Here's how the part is built. I have some questions about the finished solid (model axes, mm). Coordinates: 2 decimals unless noted, no trailing zeros. Write each loop counter-clockwise with the first axis right and the second up, starting at its lowest first coordinate (ties: lowest second). Pieces come first, ordered by that corner, then holes. Notation, with made-up numbers: (35, -17) -> (87, -17) arc R24 ccw to (87, 15) -> close; hole circle Ø5 at (83.5, 9). An arc over 180 degrees is marked (long way). Put each result on its own line as item: value.
```python
from build123d import *

# Parameters (mm, degrees)
SKETCH1_W           = 28
SKETCH1_H           = 18
BOSS_EXTRUDE2_DEPTH = 1.6
SKETCH4_R           = 0.9
CUT_EXTRUDE5_DEPTH  = 1.6
SKETCH9_R           = 0.4
CUT_EXTRUDE6_DEPTH  = 10


with BuildPart() as part:
    # Sketch1 → Boss-Extrude2 (new body)
    with BuildSketch(Plane(origin=(0, 0, 0), x_dir=(1, 0, 0), z_dir=(0, 1, 0))):
        with Locations((17.78, 7.62)):
            Rectangle(SKETCH1_W, SKETCH1_H)
    extrude(amount=BOSS_EXTRUDE2_DEPTH)

    # Sketch4 → Cut-Extrude5 (cut)
    with BuildSketch(Plane(origin=(0, 0, 0), x_dir=(1, 0, 0), z_dir=(0, 1, 0))):
        with Locations((29.76, 15.24)):
            Circle(SKETCH4_R)
        with Locations((29.76, 0)):
            Circle(SKETCH4_R)
        with Locations((6.32, 0)):
            Circle(SKETCH4_R)
        with Locations((6.32, 15.24)):
            Circle(SKETCH4_R)
    extrude(amount=CUT_EXTRUDE5_DEPTH, mode=Mode.SUBTRACT)

    # Sketch9 → Cut-Extrude6 (cut)
    with BuildSketch(Plane(origin=(0, 0, 0), x_dir=(1, 0, 0), z_dir=(0, 1, 0))):
        with Locations((27.73, 5.42)):
            Circle(SKETCH9_R)
        with Locations((27.73, 9.82)):
            Circle(SKETCH9_R)
    extrude(amount=CUT_EXTRUDE6_DEPTH, mode=Mode.SUBTRACT)


solid = part.part
```
Item 1: Imagine slicing it at C-C on x = 6.32. Write out the boundary of the cut face in (y, z), then the cut area to 3 significant figures.
Output:
outline: (0, -16.62) -> (1.6, -16.62) -> (1.6, -16.14) -> (0, -16.14) -> close; (0, -14.34) -> (1.6, -14.34) -> (1.6, -0.9) -> (0, -0.9) -> close; (0, 0.9) -> (1.6, 0.9) -> (1.6, 1.38) -> (0, 1.38) -> close
area: 23.0 mm²
Item 2: Imagine slicing it at D-D on z = -15.24. Write out the boundary of the cut face in (x, y).
Output:
outline: (3.78, 0) -> (5.42, 0) -> (5.42, 1.6) -> (3.78, 1.6) -> close; (7.22, 0) -> (28.86, 0) -> (28.86, 1.6) -> (7.22, 1.6) -> close; (30.66, 0) -> (31.78, 0) -> (31.78, 1.6) -> (30.66, 1.6) -> close
Item 3: Please list where these lines run through material, in increasing order: line 1 along X through (y, z) = (1.05, 0); line 2 along Z through (x, y) = (27.73, 1.1); line 3 along Z through (x, y) = (6.32, 0.55). Write a range as from..to.
Output:
line 1: x = 3.78..5.42, 7.22..28.86, 30.66..31.78
line 2: z = -16.62..-10.22, -9.42..-5.82, -5.02..1.38
line 3: z = -16.62..-16.14, -14.34..-0.9, 0.9..1.38
Item 4: Imagine slicing it at A-A on z = -9.82. Write out the boundary of the cut face in (x, y).
Output:
outline: (3.78, 0) -> (27.33, 0) -> (27.33, 1.6) -> (3.78, 1.6) -> close; (28.13, 0) -> (31.78, 0) -> (31.78, 1.6) -> (28.13, 1.6) -> close
Item 5: If we mould it in two halves opening along Z, with no side actions, what happens to faces 1 (the cylindrical face through (6.735, 0.789, -14.442)), 2 (the flat face through (18, 1, 1.38)), 3 (the cylindrical face through (27.33, 0.79, -5.44)), 4 (the flat face through (18, 1.6, -8))? For each: released by +Z, released by -Z, zero draft, split by the parting line, or undercut.
Output:
face 1: undercut
face 2: released by +Z
face 3: undercut
face 4: zero draft
Item 6: Imagine slicing it at B-B on y = 0.5. Write out the boundary of the cut face in (x, z), then the cut area to 3 significant figures.
Output:
outline: (3.78, -16.62) -> (31.78, -16.62) -> (31.78, 1.38) -> (3.78, 1.38) -> close; hole circle Ø1.8 at (6.32, -15.24); hole circle Ø1.8 at (6.32, 0); hole circle Ø0.8 at (27.73, -9.82); hole circle Ø0.8 at (27.73, -5.42); hole circle Ø1.8 at (29.76, -15.24); hole circle Ø1.8 at (29.76, 0)
area: 493 mm²
